Build history of the part. All positions in model axes, mm. A direction names the side the tool comes from. Round coordinates to 2 decimals unless told otherwise and drop trailing zeros. Write each loop counter-clockwise with the first axis right and the second up, starting at its lowest first coordinate (ties: lowest second). Pieces come first, ordered by that corner, then holes. Notation, with made-up numbers: (16.5, -34) -> (21.5, -34) arc R14 ccw to (21.5, -9) -> close; hole circle Ø11 at (-14, 70). An arc over 180 degrees is marked (long way). Return JSON: item names as keys, results as strings.
from build123d import *

# Parameters (mm, degrees)
SKETCH_1_W          = 80
SKETCH_1_H          = 80
EXTRUDE_1_DEPTH     = 10
SKETCH_2_R          = 17
EXTRUDE_2_DEPTH     = 3
SKETCH_3_R          = 5
EXTRUDE_3_DEPTH     = 29
CUT_EXTRUDE_1_DEPTH = 23
CUT_EXTRUDE_4_DEPTH = 2.5
SKETCH_7_W          = 80
SKETCH_7_H          = 80
EXTRUDE_6_DEPTH     = 32.5
SKETCH_10_R         = 40
EXTRUDE_7_DEPTH     = 115
SKETCH_11_R         = 14
EXTRUDE_8_DEPTH     = 5
SKETCH_12_R         = 2.75
CUT_EXTRUDE_5_DEPTH = 173.064668076
FILLET_1_R          = 5


with BuildPart() as part:
    # 스케치1 → 보스-돌출1 (new body)
    with BuildSketch(Plane.XY):
        Rectangle(SKETCH_1_W, SKETCH_1_H)
    extrude(amount=EXTRUDE_1_DEPTH)

    # 스케치2 → 보스-돌출2 (add)
    with BuildSketch(Plane.XY.offset(10)):
        with Locations((0, 15)):
            Circle(SKETCH_2_R)
    extrude(amount=EXTRUDE_2_DEPTH)

    # 스케치3 → 보스-돌출3 (add)
    with BuildSketch(Plane.XY.offset(13)):
        with Locations(Location((0, 15, 0), (0, 0, 180))):
            Circle(SKETCH_3_R)
    extrude(amount=EXTRUDE_3_DEPTH)

    # 스케치4 → 컷-돌출1 (cut)
    with BuildSketch(Plane.XY.offset(42)):
        Polygon((0, 17.5), (-2, 17.5), (-2, 20.912683476), (2, 20.912683476), (2, 17.5), align=None)
    extrude(amount=-CUT_EXTRUDE_1_DEPTH, mode=Mode.SUBTRACT)

    # 스케치6 → 컷-돌출4 (cut)
    with BuildSketch(Plane(origin=(0, 20, 0), x_dir=(1, 0, 0), z_dir=(0, 1, 0))):
        with BuildLine():
            Line((-2, -19), (-2, -52.407669752))
            Line((-2, -52.407669752), (2, -52.407669752))
            Line((2, -52.407669752), (2, -19))
            ThreePointArc((2, -19), (0, -17), (-2, -19))
        make_face()
    extrude(amount=-CUT_EXTRUDE_4_DEPTH, mode=Mode.SUBTRACT)

    # 스케치7 → 보스-돌출6 (add)
    with BuildSketch(Plane(origin=(0, 0, 0), x_dir=(-1, 0, 0), z_dir=(0, 0, -1))):
        Rectangle(SKETCH_7_W, SKETCH_7_H)
    extrude(amount=EXTRUDE_6_DEPTH)

    # 스케치10 → 보스-돌출7 (add)
    with BuildSketch(Plane(origin=(0, 0, -32.5), x_dir=(-1, 0, 0), z_dir=(0, 0, -1))):
        Circle(SKETCH_10_R)
    extrude(amount=EXTRUDE_7_DEPTH)

    # 스케치11 → 보스-돌출8 (add)
    with BuildSketch(Plane(origin=(0, 0, -147.5), x_dir=(-1, 0, 0), z_dir=(0, 0, -1))):
        Circle(SKETCH_11_R)
    extrude(amount=EXTRUDE_8_DEPTH)

    # 스케치12 → 컷-돌출5 (cut, through all)
    with BuildSketch(Plane.XY.offset(10)):
        with Locations((33.234018716, 33.234018716)):
            Circle(SKETCH_12_R)
        with Locations((-33.234018716, 33.234018716)):
            Circle(SKETCH_12_R)
        with Locations((-33.234018716, -33.234018716)):
            Circle(SKETCH_12_R)
        with Locations((33.234018716, -33.234018716)):
            Circle(SKETCH_12_R)
    extrude(amount=-CUT_EXTRUDE_5_DEPTH, mode=Mode.SUBTRACT)

    # 필렛1
    fillet_1_edges = [part.edges().sort_by_distance(p)[0] for p in [
        (40, -40, -11.25),
        (-40, -40, -11.25),
        (-40, 40, -11.25),
        (40, 40, -11.25),
    ]]
    fillet(fillet_1_edges, radius=FILLET_1_R)


solid = part.part
Q1. Saw through at C-C on x = -7. List the corners of the cut face in (y, z), then the cut area to 3 significant figures.
Verdict:
{"outline": "(-40, -32.5) -> (-39.38, -32.5) -> (-39.38, -147.5) -> (-12.12, -147.5) -> (-12.12, -152.5) -> (12.12, -152.5) -> (12.12, -147.5) -> (39.38, -147.5) -> (39.38, -32.5) -> (40, -32.5) -> (40, 10) -> (30.49, 10) -> (30.49, 13) -> (-0.49, 13) -> (-0.49, 10) -> (-40, 10) -> close", "area": "12,700 mm²"}
Q2. Saw through at D-D on z = -93. List the corners of the cut face in (x, y).
Verdict:
{"outline": "circle Ø80 at (0, 0)"}
Q3. Saw through at A-A on y = -24. List the corners of the cut face in (x, z).
Verdict:
{"outline": "(-40, -32.5) -> (-32, -32.5) -> (-32, -147.5) -> (32, -147.5) -> (32, -32.5) -> (40, -32.5) -> (40, 10) -> (-40, 10) -> close"}
Q4. Wall check: L1, parallel to Y at x = 35.5, z = 7.5; L2, parallel to Z at x = -34.5, y = -13.5; L3, parallel to Z at x = 30.5, y = -35.5. Give the ranges that are in metal, low to high.
Verdict:
{"L1": "y = -39.97 to -34.79, -31.68 to 31.68, 34.79 to 39.97", "L2": "z = -147.5 to 10", "L3": "z = -32.5 to 10"}
Q5. Two-plate mould, pull along X, no slides. Class faces 5 (the cylindrical face through (-12.932, -5.362, -149.965)), 6 (the flat face through (4, 11, 13)), 7 (the flat face through (0, 17.5, 30)): +X half, -X half, draft (parallel to the pull), parting line (faces both ways), or undercut.
Verdict:
{"face 5": "parting line", "face 6": "draft", "face 7": "undercut"}
Q6. Saw through at B-B on z = -20. List the corners of the cut face in (x, y), then the cut area to 3 significant figures.
Verdict:
{"outline": "(-40, -35) arc R5 ccw to (-35, -40) -> (35, -40) arc R5 ccw to (40, -35) -> (40, 35) arc R5 ccw to (35, 40) -> (-35, 40) arc R5 ccw to (-40, 35) -> close; hole circle Ø5.5 at (-33.23, -33.23); hole circle Ø5.5 at (-33.23, 33.23); hole circle Ø5.5 at (33.23, -33.23); hole circle Ø5.5 at (33.23, 33.23)", "area": "6,280 mm²"}
Q7. Pin check, flat tips, straight feed: pin 1 Ø5 at (x, y) = (4.5, 31) entering from -Z; pin 2 Ø1.5 at (x, y) = (-8, 19.5) entering from +Z; pin 3 Ø1.5 at (y, z) = (17, -77.5) entering from -X. Stop position of each tip, or through.
Verdict:
{"pin 1": "stops at z = -147.5", "pin 2": "stops at z = 13", "pin 3": "stops at x = -36.55"}
Q8. 3-axis set-ups, long thin cutter, end or side, ignore diameter. For faces 1 (the flat face through (-30, 30, -32.5)), 2 (the cylindrical face through (0.651, 10.043, 27.297)), 3 (the flat face through (1, -17, -147.5)), 4 (the flat face through (30, -32, -32.5)): which of +Z, -Z, +X, -X, +Y, -Y reach the whole face in a straight line?
Verdict:
{"face 1": "-Z, -X, +Y", "face 2": "+Z", "face 3": "-Z", "face 4": "-Z, +X, -Y"}
